For this review, take the finished solid that the model builds, in its own axes (mm). A direction names the side the tool comes from. Give positions to 0.01 mm unless a question says otherwise; leave off trailing zeros. Order: outer loops, then holes, each group sorted by start corner. A loop starts at its lowest first (then second) coordinate and runs counter-clockwise, first axis right, second up. Notation, with made-up numbers: (-32, -35) - (-20, -35) arc R22 cw to (-20, -10) - close; hole circle Ø1 at (77, -22.75). An arc over 180 degrees is marked (long way). Put each result on its own line as item: value. Start each with the question number.
```python
from build123d import *

# Parameters (mm, degrees)
SKETCH2_W           = 100
SKETCH2_H           = 100
BOSS_EXTRUDE1_DEPTH = 2.5
BOSS_EXTRUDE2_DEPTH = 27.5
SKETCH9_W           = 32
SKETCH9_H           = 52.5
CUT_EXTRUDE3_DEPTH  = 2.5
CUT_EXTRUDE4_REACH  = 117.758
SKETCH5_W           = 40
SKETCH5_H           = 30


with BuildPart() as part:
    # Sketch2 → Boss-Extrude1 (new body)
    with BuildSketch(Plane(origin=(0, 0, 0), x_dir=(1, 0, 0), z_dir=(0, 1, 0))):
        Rectangle(SKETCH2_W, SKETCH2_H)
    extrude(amount=BOSS_EXTRUDE1_DEPTH)

    # Sketch4 → Boss-Extrude2 (add)
    with BuildSketch(Plane(origin=(0, 2.5, 0), x_dir=(1, 0, 0), z_dir=(0, 1, 0))):
        Polygon((-50, 50), (-50, -50), (50, -50), (50, 50), (16, 50), (16, 47.5), (16, -2.5), (-16, -2.5), (-16, 47.5), (-16, 50), align=None)
        Polygon((-47.5, -47.5), (47.5, -47.5), (47.5, -32.25), (22.5, -32.25), (22.5, -29.75), (47.5, -29.75), (47.5, -17.75), (22.5, -17.75), (22.5, -15.25), (47.5, -15.25), (47.5, 47.5), (18.5, 47.5), (18.5, -5), (-18.5, -5), (-18.5, 47.5), (-47.5, 47.5), (-47.5, -15.25), (-22.5, -15.25), (-22.5, -17.75), (-47.5, -17.75), (-47.5, -29.75), (-22.5, -29.75), (-22.5, -32.25), (-47.5, -32.25), align=None, mode=Mode.SUBTRACT)
    extrude(amount=BOSS_EXTRUDE2_DEPTH)

    # Sketch9 → Cut-Extrude3 (cut)
    with BuildSketch(Plane(origin=(0, 2.5, 0), x_dir=(1, 0, 0), z_dir=(0, 1, 0))):
        with Locations((0, 23.75)):
            Rectangle(SKETCH9_W, SKETCH9_H)
    extrude(amount=-CUT_EXTRUDE3_DEPTH, mode=Mode.SUBTRACT)

    # Cut-Extrude4: up to this face of the body (flat: up to its plane)
    cut_extrude4_end = Plane(part.part.faces().sort_by_distance((-50, 15, 0))[0])
    # Sketch5 → Cut-Extrude4 (cut, up to the picked face)
    with BuildSketch(Plane(origin=(50, 0, 0), x_dir=(0, 0, -1), z_dir=(1, 0, 0)), mode=Mode.PRIVATE) as cut_extrude4_sk1:
        with Locations((30, 15)):
            Rectangle(SKETCH5_W, SKETCH5_H)
    cut_extrude4_tool1 = split(extrude(cut_extrude4_sk1.sketch, amount=-CUT_EXTRUDE4_REACH, mode=Mode.PRIVATE), bisect_by=cut_extrude4_end, keep=Keep.BOTH, mode=Mode.PRIVATE)
    add(cut_extrude4_tool1.solids().sort_by(Axis((50, 15, -30), (-1, 0, 0)))[0], mode=Mode.SUBTRACT)


solid = part.part
```
1. Clearance check with flat-ended pins moving along their axes: pin 1 (7.5 mm diameter, centred on x = 37.5, y = 22, fed in from -Z); pin 2 (6 mm diameter, centred on x = -30.5, y = 3.5, fed in from -Z); pin 3 (6 mm diameter, centred on x = 26, z = -1, fed in from +Y); pin 4 (9 mm diameter, centred on x = -7.5, y = 9, fed in from -Z). State where each tip first meets the part, or that it passes through.
2. The part is to be moulded in two halves that separate along X. For faces 4 (the face through (-50, 15, 20)), 5 (the face through (-1, 0, 20)), 6 (the face through (-35, 16, 32.25)), say which applies: released by +X, released by -X, zero draft, split by the parting line, or undercut.
3. Add section C-C, the plane x = 30. Give the boundary of the cut face in (y, z).
4. Add section B-B, the plane z = -1. Give the boundary of the cut face in (x, y), then the cut area to 3 significant figures.
5. Add section D-D, the plane z = 19.5. Give the boundary of the cut face in (x, y).
6. Wall thickness on line 1 (Z direction, x = -37, y = 26.5); line 2 (X direction, y = 20, z = 4.5); line 3 (X direction, y = 6, z = -4.5): over which ranges is each line inside the solid? List them lowest first. Write a range as from..to.
7. Tool access review of faces 1 (the face through (16, 15, -4)), 2 (the face through (-22.5, 16, 31)), 3 (the face through (0, 16, 5)): name each direction out of +Z, -Z, +X, -X, +Y, -Y from which nothing blocks a thin tool from reaching the whole face with its end or side.
Found:
1. pin 1: stops at z = 15.25
1. pin 2: stops at z = -10
1. pin 3: stops at y = 2.5
1. pin 4: stops at z = 2.5
2. face 4: released by -X
2. face 5: zero draft
2. face 6: undercut
3. outline: (0, -10) - (2.5, -10) - (2.5, 15.25) - (30, 15.25) - (30, 17.75) - (2.5, 17.75) - (2.5, 29.75) - (30, 29.75) - (30, 32.25) - (2.5, 32.25) - (2.5, 47.5) - (30, 47.5) - (30, 50) - (0, 50) - close
4. outline: (-50, 0) - (-16, 0) - (-16, 30) - (-18.5, 30) - (-18.5, 2.5) - (-47.5, 2.5) - (-47.5, 30) - (-50, 30) - close; (16, 0) - (50, 0) - (50, 30) - (47.5, 30) - (47.5, 2.5) - (18.5, 2.5) - (18.5, 30) - (16, 30) - close
4. area: 445 mm^2
5. outline: (-50, 0) - (50, 0) - (50, 30) - (47.5, 30) - (47.5, 2.5) - (-47.5, 2.5) - (-47.5, 30) - (-50, 30) - close
6. line 1: z = 15.25..17.75, 29.75..32.25, 47.5..50
6. line 2: x = -50..-47.5, -18.5..18.5, 47.5..50
6. line 3: x = -50..-47.5, -18.5..-16, 16..18.5, 47.5..50
7. face 1: -Z, +Y, -Y
7. face 2: -Z, +Y
7. face 3: +Y
